Here's how the part is built. I have some questions about the finished solid (model axes, mm). Face numbers are marked on the shaded views. A direction names the side the tool comes from. Round coordinates to 2 decimals unless told otherwise and drop trailing zeros. Write each loop counter-clockwise with the first axis right and the second up, starting at its lowest first coordinate (ties: lowest second). Pieces come first, ordered by that corner, then holes. Notation, with made-up numbers: (4, -20) -> (32, -20) arc R30 cw to (32, 16) -> close; hole circle Ø7 at (-39.75, -11). An arc over 180 degrees is marked (long way). Answer as CSV lines item,"result".
```python
from build123d import *

# Parameters (mm, degrees)
F0_R     = 30
F0_R_2   = 10
F1_DEPTH = 15
F2_R     = 5
F3_DEPTH = 1.5
F4_R     = 25
F4_R_2   = 15
F5_DEPTH = 10
F7_D     = 4
F7_DEPTH = 45
F7_TIP   = 1.2017212381
F8_R     = 1


with BuildPart() as f1:
    # F0 (on Front) → F1 (new body)
    with BuildSketch(Plane.XZ):
        with Locations((0, -30.0189442933)):
            Circle(F0_R)
        with Locations((0, -30.0189442933)):
            Circle(F0_R_2, mode=Mode.SUBTRACT)
    extrude(amount=F1_DEPTH)

    # F2 (on Top) → F3 (cut)
    with BuildSketch(Plane.XY):
        with Locations((0, -9)):
            Circle(F2_R)
    extrude(amount=-F3_DEPTH, mode=Mode.SUBTRACT)

    # F4 (on face) → F5 (cut)
    with BuildSketch(Plane.XZ.offset(15)):
        with Locations((0, -30.0189442933)):
            Circle(F4_R)
        with Locations((0, -30.0189442933)):
            Circle(F4_R_2, mode=Mode.SUBTRACT)
    extrude(amount=-F5_DEPTH, mode=Mode.SUBTRACT)

    # F7
    with Locations(Plane.XY):
        with Locations((0, -9)):
            Hole(F7_D / 2, depth=F7_DEPTH)
            with Locations((0, 0, -(F7_DEPTH + F7_TIP / 2))):  # 118° drill point
                Cone(0, F7_D / 2, F7_TIP, mode=Mode.SUBTRACT)

    # F8
    f8_edges = [f1.edges().sort_by_distance(p)[0] for p in [
        (-10, 0, -30.018944),
        (-10, -15, -30.018944),
    ]]
    fillet(f8_edges, radius=F8_R)


solid = f1.part
```
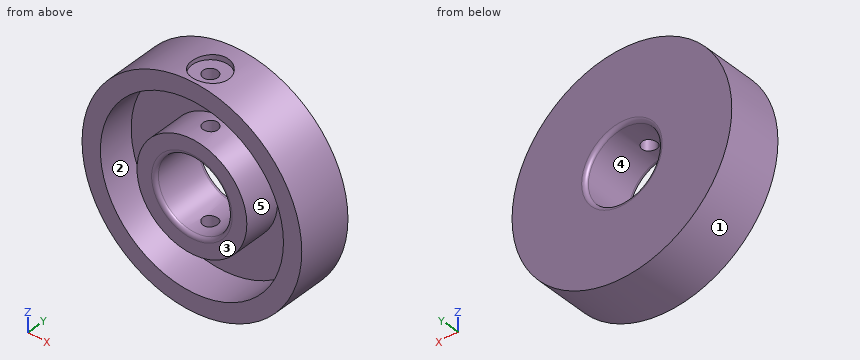
1. On a 3-axis mill with a long thin cutter (end or side, diameter ignored), from which of +Z, -Z, +X, -X, +Y, -Y can I reach the whole of each face in a straight line? I mean the marked faces 4 and 5. Say none if no direction works.
Numbers:
face 4,"+Y, -Y"
face 5,"-Y"
2. Suppose I cut it at D-D on z = -42. Please give me the cut outline in (x, y).
Numbers:
outline,"(-27.5, -15) -> (-21.94, -15) -> (-21.94, -5) -> (-9.03, -5) -> (-9.03, -15) -> (9.03, -15) -> (9.03, -5) -> (21.94, -5) -> (21.94, -15) -> (27.5, -15) -> (27.5, 0) -> (-27.5, 0) -> close; hole circle Ø4 at (0, -9)"
3. Suppose I cut it at A-A on y = -12.25. Please give me the cut outline in (x, z).
Numbers:
outline,"circle Ø30 at (0, -30.02); (-3.8, -1.5) -> (-3.8, -0.26) arc R30 ccw (long way) to (3.8, -0.26) -> (3.8, -1.5) -> close; hole circle Ø50 at (0, -30.02); hole circle Ø20 at (0, -30.02)"
4. Suppose I cut it at C-C on x = 24. Please give me the cut outline in (y, z), and give its area (3 significant figures).
Numbers:
outline,"(-15, -48.02) -> (0, -48.02) -> (0, -12.02) -> (-15, -12.02) -> (-15, -23.02) -> (-5, -23.02) -> (-5, -37.02) -> (-15, -37.02) -> close"
area,"400 mm^2"
5. If I drill on line 1 (X direction, y = -9, z = -17.8); line 2 (Y direction, x = 0, z = -16); line 3 (Z direction, x = 12, y = -8), over which ranges is the centre line in solid material (lowest first)?
Numbers:
line 1,"x = -27.4 to -21.81, -8.7 to -2, 2 to 8.7, 21.81 to 27.4"
line 2,"y = -15 to -11, -7 to 0"
line 3,"z = -57.51 to -51.95, -39.02 to -21.02, -8.09 to -2.52"
6. Suppose I cut it at B-B on y = -9. Please give me the cut outline in (x, z).
Numbers:
outline,"(-5, -1.5) -> (-5, -0.44) arc R30 ccw (long way) to (5, -0.44) -> (5, -1.5) -> (2, -1.5) -> (2, -5.1) arc R25 cw (long way) to (-2, -5.1) -> (-2, -1.5) -> close; (-2, -44.89) -> (-2, -39.82) arc R10 cw to (-2, -20.22) -> (-2, -15.15) arc R15 ccw to start; (2, -44.89) arc R15 ccw to (2, -15.15) -> (2, -20.22) arc R10 cw to (2, -39.82) -> close"
7. If we mould it in two halves opening along X, with no side actions, what happens to the marked faces 1, 2 and 3? For each: released by +X, released by -X, zero draft, split by the parting line, or undercut.
Numbers:
face 1,"split by the parting line"
face 2,"undercut"
face 3,"zero draft"
8. For pin 1 Ø2 at (x, z) = (2, -14) entering from -Y; pin 2 Ø5 at (x, y) = (18, -11) entering from +Z; pin 3 Ø3 at (x, y) = (0, -9) entering from -Z; pin 4 Ø5 at (y, z) = (-8.5, -28.5) entering from -X, each with a flat end and sliding along its axis, tell me the tip position at first contact or that it passes through.
Numbers:
pin 1,"stops at y = -5"
pin 2,"stops at z = -4.33"
pin 3,"stops at z = -60.02"
pin 4,"stops at x = -30"
